For this review, take the finished solid that the model builds, in its own axes (mm). Face numbers are marked on the shaded views. Coordinates: 2 decimals unless noted, no trailing zeros. Loops run counter-clockwise (first coordinate to the right, second up) from the corner with the lowest first, then second, coordinate; pieces in that order, holes last. Notation, with made-up numbers: (41.25, -37) -> (49.25, -37) arc R3 cw to (49.25, -32) -> close; hole circle Ø6 at (-15, 9.25). An arc over 180 degrees is marked (long way). Answer in a Markdown table with one row per item.
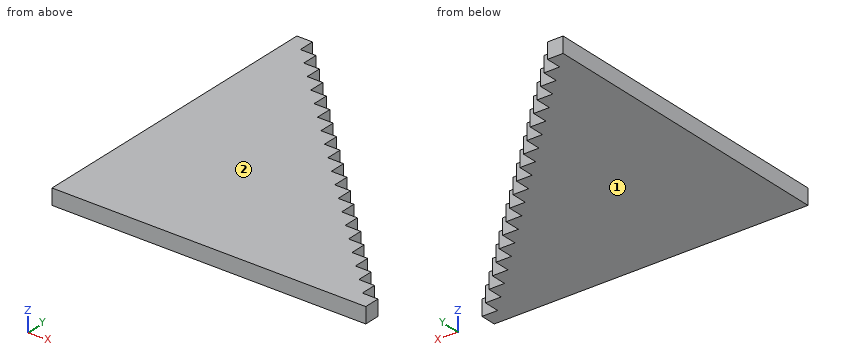
from build123d import *

# Parameters (mm, degrees)
BOSS_EXTRUDE1_DEPTH = 2


with BuildPart() as part:
    # Sketch1 → Boss-Extrude1 (new body)
    with BuildSketch(Plane.XY):
        Polygon((-79.033423275, -42.190980898), (-77.033423275, -42.190980898), (-77.033423275, -44.190980898), (-75.033423275, -44.190980898), (-75.033423275, -46.190980898), (-73.033423275, -46.190980898), (-73.033423275, -48.190980898), (-71.033423275, -48.190980898), (-71.033423275, -50.190980898), (-69.033423275, -50.190980898), (-69.033423275, -52.190980898), (-67.033423275, -52.190980898), (-67.033423275, -54.190980898), (-65.033423275, -54.190980898), (-65.033423275, -56.190980898), (-63.033423275, -56.190980898), (-63.033423275, -58.190980898), (-61.033423275, -58.190980898), (-61.033423275, -60.190980898), (-59.033423275, -60.190980898), (-59.033423275, -62.190980898), (-57.033423275, -62.190980898), (-57.033423275, -64.190980898), (-55.033423275, -64.190980898), (-55.033423275, -66.190980898), (-53.033423275, -66.190980898), (-53.033423275, -68.190980898), (-51.033423275, -68.190980898), (-51.033423275, -70.190980898), (-49.033423275, -70.190980898), (-49.033423275, -72.190980898), (-47.033423275, -72.190980898), (-47.033423275, -74.190980898), (-45.033423275, -74.190980898), (-45.033423275, -76.190980898), (-43.033423275, -76.190980898), (-43.033423275, -78.190980898), (-41.033423275, -78.190980898), (-41.033423275, -80.190980898), (-39.033423275, -80.190980898), (-39.033423275, -82.190980898), (-79.033423275, -82.190980898), (-79.033423275, -80.190980898), (-79.033423275, -78.190980898), (-79.033423275, -76.190980898), (-79.033423275, -74.190980898), (-79.033423275, -72.190980898), (-79.033423275, -70.190980898), (-79.033423275, -68.190980898), (-79.033423275, -66.190980898), (-79.033423275, -64.190980898), (-79.033423275, -62.190980898), (-79.033423275, -60.190980898), (-79.033423275, -58.190980898), (-79.033423275, -56.190980898), (-79.033423275, -54.190980898), (-79.033423275, -52.190980898), (-79.033423275, -50.190980898), (-79.033423275, -48.190980898), (-79.033423275, -46.190980898), (-79.033423275, -44.190980898), align=None)
    extrude(amount=BOSS_EXTRUDE1_DEPTH)


solid = part.part
Item 1: Take a section at B-B, the plane x = -70.5. State the section outline as (y, z) points, and give its area (3 significant figures).
Worked answers:
| item | result |
|---|---|
| outline | (-82.19, 0) -> (-50.19, 0) -> (-50.19, 2) -> (-82.19, 2) -> close |
| area | 64.0 mm² |
Item 2: Insertion check: pin 1 (0.6 mm diameter, centred on x = -66, z = 0.5, fed in from +Y); pin 2 (1 mm diameter, centred on y = -55, z = 1, fed in from +X); pin 3 (1 mm diameter, centred on y = -79, z = 1, fed in from +X). Each pin has a flat end and moves straight along its axis. Give the tip position at first contact, or say it passes through.
Worked answers:
| item | result |
|---|---|
| pin 1 | y = -54.19 |
| pin 2 | x = -65.03 |
| pin 3 | x = -41.03 |
Item 3: The part is to be moulded in two halves that separate along Z. For the marked faces 1 and 2, say which applies: +Z half, -Z half, draft (parallel to the pull), parting line (faces both ways), or undercut.
Worked answers:
| item | result |
|---|---|
| face 1 | -Z half |
| face 2 | +Z half |
Item 4: Take a section at A-A, the plane y = -63. State the section outline as (x, z) points.
Worked answers:
| item | result |
|---|---|
| outline | (-79.03, 0) -> (-57.03, 0) -> (-57.03, 2) -> (-79.03, 2) -> close |
Item 5: For L1, parallel to X at y = -45.5, z = 0.25; L2, parallel to Y at x = -67, z = 1.4; L3, parallel to Y at x = -65, z = 0.5, list the stretches that pass through material, from the lowest coordinate up.
Worked answers:
| item | result |
|---|---|
| L1 | -79.03 to -75.03 |
| L2 | -82.19 to -54.19 |
| L3 | -82.19 to -56.19 |
